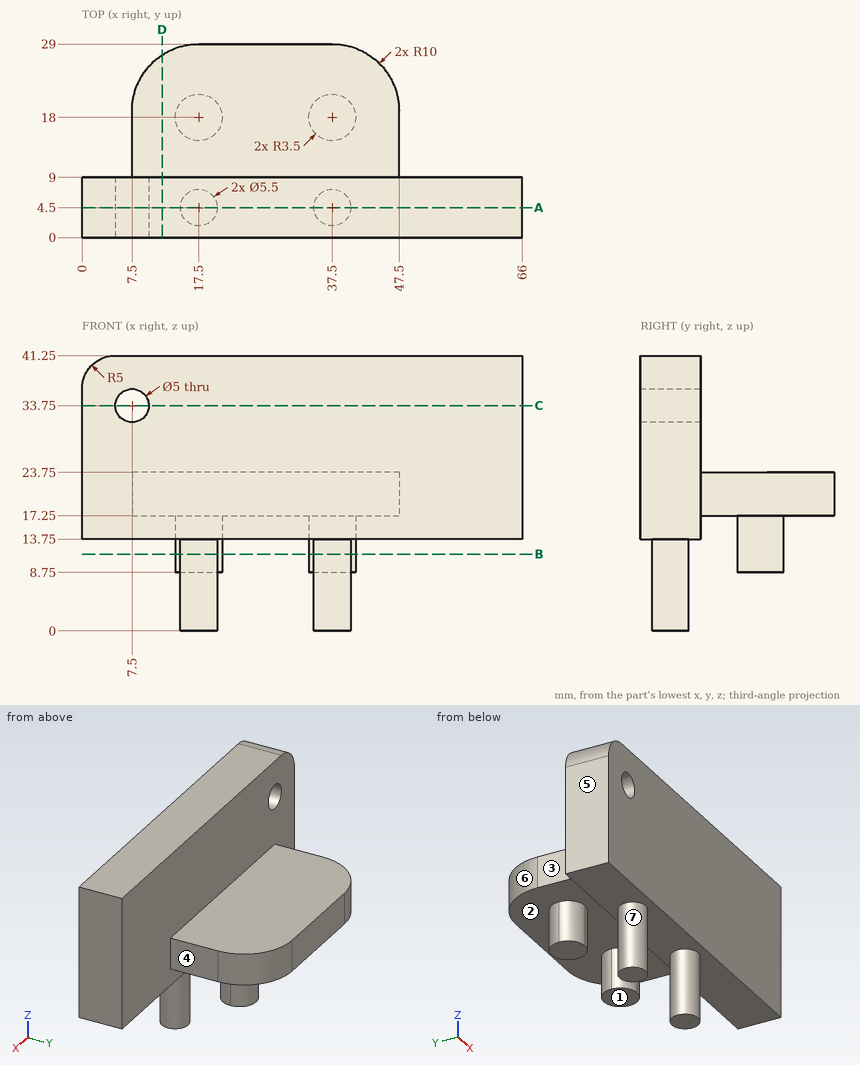
For this review, use the dimensioned drawing (mm, ordinates from the lowest corner) and the shaded views. A direction names the side the tool comes from. Round coordinates to 2 decimals unless told otherwise and drop trailing zeros. Write each loop counter-clockwise with the first axis right and the second up, starting at its lowest first coordinate (ties: lowest second). Pieces come first, ordered by that corner, then holes. Notation, with made-up numbers: (49, 13.25) - (61, 13.25) arc R19 ccw to (61, 47.25) - close; hole circle Ø5 at (32, -37). An arc over 180 degrees is marked (long way). Answer as a JSON object with one key per item and string values.
1. Draft analysis for pull direction Y (two halves, no side actions). For the marked faces 5, 6 and 7, state which applies: +Y half, -Y half, draft (parallel to the pull), parting line (faces both ways), or undercut.
Response values:
{"face 5": "draft", "face 6": "+Y half", "face 7": "undercut"}
2. We need section B-B on z = 11.5. Give the boundary of the cut face in (x, y), then the cut area to 3 significant figures.
Response values:
{"outline": "circle Ø7 at (17.5, 18); circle Ø5.5 at (17.5, 4.5); circle Ø7 at (37.5, 18); circle Ø5.5 at (37.5, 4.5)", "area": "124 mm2"}
3. We need section D-D on x = 12. Give the boundary of the cut face in (y, z).
Response values:
{"outline": "(0, 13.75) - (9, 13.75) - (9, 17.25) - (27.35, 17.25) - (27.35, 23.75) - (9, 23.75) - (9, 41.25) - (0, 41.25) - close"}
4. Tool access review of the marked faces 1, 2, 3 and 4: name each direction out of +Z, -Z, +X, -X, +Y, -Y from which nothing blocks a thin tool from reaching the whole face with its end or side.
Response values:
{"face 1": "-Z, +X, -X, +Y", "face 2": "-Z", "face 3": "+Z, -Z, -X, +Y", "face 4": "+Z, -Z, +X, +Y"}
5. To check wall thickness, follow line 1 along X through (y, z) = (5.5, 33.75); line 2 along Y through (x, z) = (15.5, 25); line 3 along Z through (x, y) = (17.5, 18.5). State the ranges of each line that lie inside material, in increasing order.
Response values:
{"line 1": "x = 0 to 5, 10 to 66", "line 2": "y = 0 to 9", "line 3": "z = 8.75 to 23.75"}
6. We need section A-A on y = 4.5. Give the boundary of the cut face in (x, z).
Response values:
{"outline": "(0, 13.75) - (14.75, 13.75) - (14.75, 0) - (20.25, 0) - (20.25, 13.75) - (34.75, 13.75) - (34.75, 0) - (40.25, 0) - (40.25, 13.75) - (66, 13.75) - (66, 41.25) - (5, 41.25) arc R5 ccw to (0, 36.25) - close; hole circle Ø5 at (7.5, 33.75)"}
7. For pin 1 Ø4.5 at (x, y) = (42, 3.5) entering from -Z; pin 2 Ø3 at (x, z) = (20, 34.5) entering from +Y; pin 3 Ø2 at (y, z) = (17.5, 17) entering from +X; pin 4 Ø5 at (y, z) = (13, 7.5) entering from -X, all flat-tipped, find the tip position at first contact; note any pin that passes through.
Response values:
{"pin 1": "stops at z = 0", "pin 2": "stops at y = 9", "pin 3": "stops at x = 47.5", "pin 4": "stops at x = 15.45"}
8. We need section C-C on z = 33.75. Give the boundary of the cut face in (x, y), then the cut area to 3 significant figures.
Response values:
{"outline": "(0, 0) - (5, 0) - (5, 9) - (0, 9) - close; (10, 0) - (66, 0) - (66, 9) - (10, 9) - close", "area": "549 mm2"}
